from build123d import *

# Parameters (mm, degrees)
SKETCH1_W           = 44.45
SKETCH1_H           = 44.45
BOSS_EXTRUDE1_DEPTH = 19.05


with BuildPart() as part:
    # Sketch1 → Boss-Extrude1 (new body)
    with BuildSketch(Plane(origin=(0, 0, 0), x_dir=(1, 0, 0), z_dir=(0, 1, 0))):
        Polygon((-86.995, 86.995), (-104.775, 86.995), (-104.775, -86.995), (-86.995, -86.995), (-86.995, -104.775), (86.995, -104.775), (86.995, -86.995), (104.775, -86.995), (104.775, 86.995), (86.995, 86.995), (86.995, 104.775), (-86.995, 104.775), align=None)
        Rectangle(SKETCH1_W, SKETCH1_H, mode=Mode.SUBTRACT)
    extrude(amount=BOSS_EXTRUDE1_DEPTH)


solid = part.part
Could you check a few things on this model? Use its own coordinates, in mm. A direction names the side the tool comes from. Give positions to 0.01 mm unless a question says otherwise; leave off trailing zeros. Order: outer loops, then holes, each group sorted by start corner. A loop starts at its lowest first (then second) coordinate and runs counter-clockwise, first axis right, second up.
1. Suppose I cut it at A-A (z = -17.5). List the corners of the cut face in (x, y) for me (3 decimals).
2. Suppose I cut it at B-B (y = 15.5). List the corners of the cut face in (x, z) for me (3 decimals).
3. For faces 5 (the flat face through (-86.995, 9, 96)), 6 (the flat face through (86.995, 9, -96)), 7 (the flat face through (-86.995, 9, -96)), 8 (the flat face through (0, 9, 22.225)), 9 (the flat face through (96, 9, 86.995)), which set-ups out of +Z, -Z, +X, -X, +Y, -Y let a thin tool reach every point of the face, with its end or its side?
4. We'd pull the mould along Z, two halves only. Please class faces 1 (the flat face through (22.225, 9, 0)), 2 (the flat face through (-96, 9, -86.995)), 3 (the flat face through (-22.225, 9, 0)), 4 (the flat face through (-25, 19.05, -1)): pulls with the +Z half, pulls with the -Z half, needs draft (parallel to the pull), parting line crosses it, or undercut.
5. Will these pins go through, and if not, where does the flat tip stop? P1, Ø6, axis at x = -78, z = 80.5, coming from the -Y side; P2, Ø9, axis at y = 13.5, z = -98.5, coming from the -X side (3 decimals); P3, Ø5.5, axis at x = 95, y = 11, coming from the -Z side (3 decimals); P4, Ø9, axis at x = -98, y = 5, coming from the +Z side (3 decimals).
6. I need wall thicknesses on L1, parallel to X at y = 17.5, z = 9.5 (3 decimals); L2, parallel to X at y = 14.5, z = 94 (3 decimals). Which ranges of each line are inside material? Lowest first, please.
Solved:
1. outline: (-104.775, 0) - (-22.225, 0) - (-22.225, 19.05) - (-104.775, 19.05) - close; (22.225, 0) - (104.775, 0) - (104.775, 19.05) - (22.225, 19.05) - close
2. outline: (-104.775, -86.995) - (-86.995, -86.995) - (-86.995, -104.775) - (86.995, -104.775) - (86.995, -86.995) - (104.775, -86.995) - (104.775, 86.995) - (86.995, 86.995) - (86.995, 104.775) - (-86.995, 104.775) - (-86.995, 86.995) - (-104.775, 86.995) - close; hole (-22.225, -22.225) - (22.225, -22.225) - (22.225, 22.225) - (-22.225, 22.225) - close
3. face 5: +Z, -X, +Y, -Y
3. face 6: -Z, +X, +Y, -Y
3. face 7: -Z, -X, +Y, -Y
3. face 8: +Y, -Y
3. face 9: +Z, +X, +Y, -Y
4. face 1: undercut
4. face 2: pulls with the -Z half
4. face 3: undercut
4. face 4: needs draft
5. P1: stops at y = 0
5. P2: stops at x = -86.995
5. P3: stops at z = -86.995
5. P4: stops at z = 86.995
6. L1: x = -104.775 to -22.225, 22.225 to 104.775
6. L2: x = -86.995 to 86.995
